Check sheet for the drawn part. Datum: minimum x, y, z corner. Units: mm. Coordinates: 2 decimals unless noted, no trailing zeros. Write each loop counter-clockwise with the first axis right and the second up, starting at its lowest first coordinate (ties: lowest second). Pieces come first, ordered by that corner, then holes. Notation, with made-up numbers: (-17.5, 67) - (32.5, 67) arc R7 cw to (32.5, 80) - close; hole circle Ø11 at (46, -32.75). An arc over 180 degrees is marked (long way). Use CSV: the item, a comma, the result in double quotes. Start each with the question number.
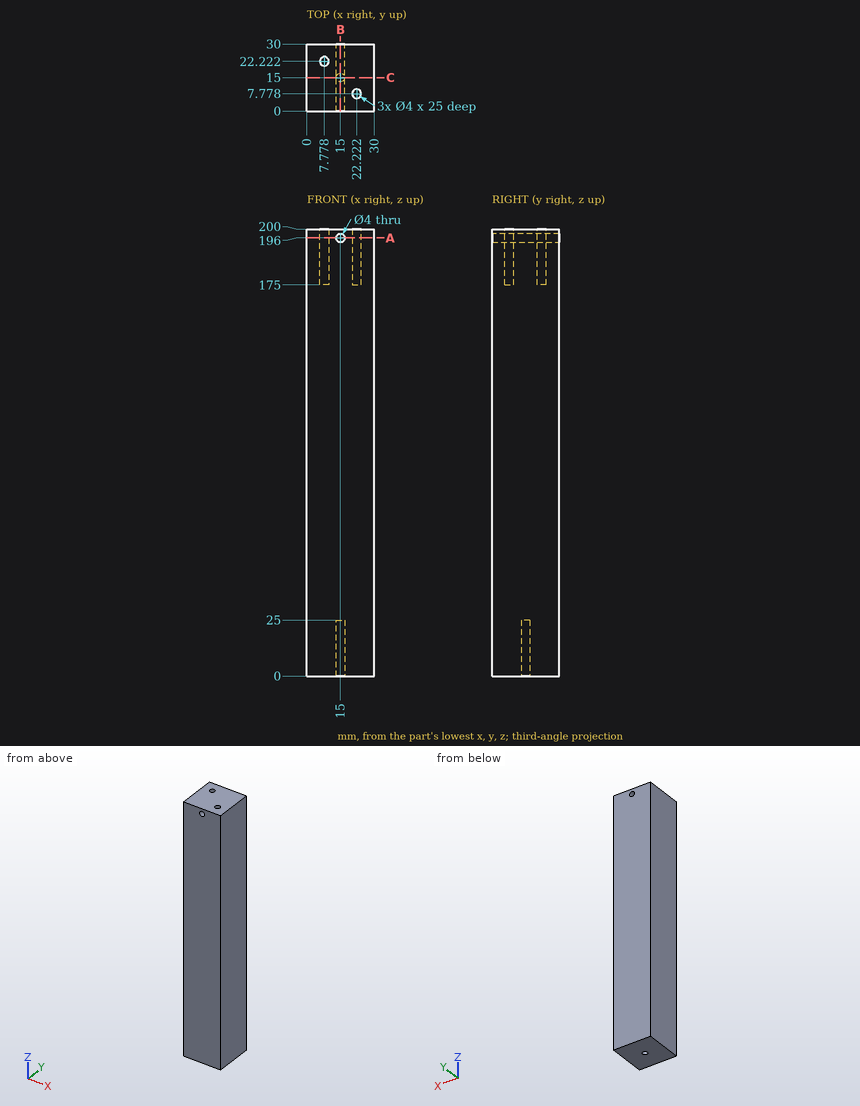
Q1. Cross-section at C-C (y = 15). Record the cut outline in (x, z).
Q2. Cross-section at A-A (z = 196). Record the cut outline in (x, y).
Q3. Cross-section at B-B (x = 15). Record the cut outline in (y, z), plus the area to 3 significant figures.
Q4. Scan lines: line 1 along X through (y, z) = (8, 196); line 2 along Z through (x, y) = (15.75, 25); line 3 along X through (y, z) = (13.5, 196). Record each from-to range of solid material in increasing order. Write a range as from..to.
Q5. Gauge pin test, flat end, axial feed: pin 1 (3 mm diameter, centred on x = 8, y = 22.5, fed in from +Z). Record the tip position at first contact, or that the pin passes through.
Reply:
1,outline,"(0, 0) - (13, 0) - (13, 25) - (17, 25) - (17, 0) - (30, 0) - (30, 200) - (0, 200) - close; hole circle Ø4 at (15, 196)"
2,outline,"(0, 0) - (13, 0) - (13, 30) - (0, 30) - close; (17, 0) - (30, 0) - (30, 30) - (17, 30) - close; hole circle Ø4 at (7.78, 22.22); hole circle Ø4 at (22.22, 7.78)"
3,outline,"(0, 0) - (13, 0) - (13, 25) - (17, 25) - (17, 0) - (30, 0) - (30, 194) - (0, 194) - close; (0, 198) - (30, 198) - (30, 200) - (0, 200) - close"
3,area,"5,780 mm^2"
4,line 1,"0..13, 17..20.23, 24.21..30"
4,line 2,"0..194.15, 197.85..200"
4,line 3,"0..13, 17..30"
5,pin 1,"z = 175"
